```python
from build123d import *

# Parameters (mm, degrees)
F0_W     = 10
F0_H     = 13
F1_DEPTH = 32
F2_R     = 5.5
F3_DEPTH = 25
F4_R     = 6.5
F5_DEPTH = 25
F7_DEPTH = 19


with BuildPart() as f1:
    # F0 (on Front) → F1 (new body)
    with BuildSketch(Plane.XZ):
        with Locations((-52.5, -6.5)):
            Rectangle(F0_W, F0_H)
        Polygon((-47.5, 0), (-47.5, -13), (-18.5, -13), (-18.5, 0), (0, 0), (0, 13), (-13.5, 13), (-13.5, 51), (-32.5, 51), (-32.5, 0), align=None)
    extrude(amount=-F1_DEPTH)

    # F2 (on face) → F3 (cut)
    with BuildSketch(Plane.XY):
        with Locations((-45, 19)):
            Circle(F2_R)
        Polygon((-57.5, 0), (-47.5, 0), (-57.5, 10), align=None)
    extrude(amount=-F3_DEPTH, mode=Mode.SUBTRACT)

    # F4 (on face) → F5 (cut)
    with BuildSketch(Plane.YZ.offset(-13.5)):
        with Locations((16, 33)):
            Circle(F4_R)
    extrude(amount=-F5_DEPTH, mode=Mode.SUBTRACT)

    # F6 (on face) → F7 (join)
    with BuildSketch(Plane.YZ.offset(-13.5)):
        with BuildLine():
            Line((0, 51), (32, 51))
            ThreePointArc((32, 51), (16, 54.871235), (0, 51))
        make_face()
    extrude(amount=-F7_DEPTH)

    # F8: F1 across plane


with BuildPart() as f1_1:
    add(f1.part)
    add(f1.part.mirror(Plane.YZ))


solid = f1_1.part
```
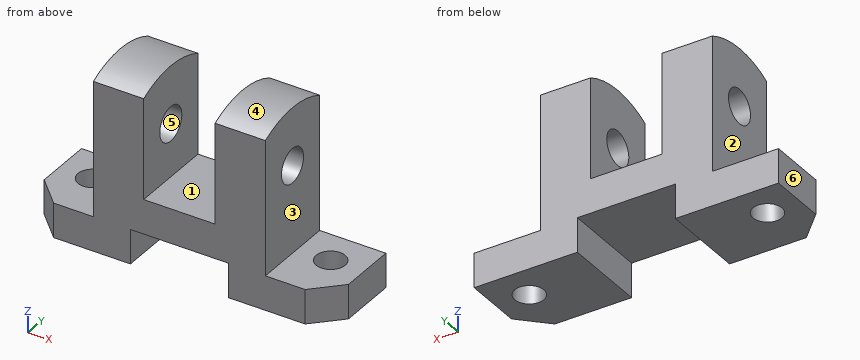
Could you check a few things on this model? Use its own coordinates, in mm. Face numbers are marked on the shaded views. A direction names the side the tool comes from. Coordinates: 2 decimals unless noted, no trailing zeros. Write each loop counter-clockwise with the first axis right and the second up, starting at its lowest first coordinate (ties: lowest second). Pieces come first, ordered by that corner, then holes. Notation, with made-up numbers: (35, -8) - (91, -8) arc R13 ccw to (91, 7) - close; hole circle Ø9 at (-34, 58). An arc over 180 degrees is marked (long way). Use a Markdown table: item, result.
Q1. Imagine slicing it at A-A (z = 33). List the corners of the cut face in (x, y) for me, and give its area (3 significant figures).
Geometry check:
| item | result |
|---|---|
| outline | (-32.5, 0) - (-13.5, 0) - (-13.5, 9.5) - (-32.5, 9.5) - close; (-32.5, 22.5) - (-13.5, 22.5) - (-13.5, 32) - (-32.5, 32) - close; (13.5, 0) - (32.5, 0) - (32.5, 9.5) - (13.5, 9.5) - close; (13.5, 22.5) - (32.5, 22.5) - (32.5, 32) - (13.5, 32) - close |
| area | 722 mm2 |
Q2. I'm going to push flat-ended pins straight in: pin 1 Ø17.5 at (x, y) = (45, 19) entering from +Z; pin 2 Ø13.5 at (x, y) = (6, 15) entering from +Z; pin 3 Ø16 at (y, z) = (19, 35) entering from +X. Where does each tip first touch, or does it pass through?
Geometry check:
| item | result |
|---|---|
| pin 1 | stops at z = 0 |
| pin 2 | stops at z = 13 |
| pin 3 | stops at x = 32.5 |
Q3. Imagine slicing it at D-D (x = 20.5). List the corners of the cut face in (y, z) for me, and give its area (3 significant figures).
Geometry check:
| item | result |
|---|---|
| outline | (0, -13) - (32, -13) - (32, 51) arc R35 ccw to (0, 51) - close; hole circle Ø13 at (16, 33) |
| area | 2,000 mm2 |
Q4. Imagine slicing it at B-B (x = -45). List the corners of the cut face in (y, z) for me, and give its area (3 significant figures).
Geometry check:
| item | result |
|---|---|
| outline | (0, -13) - (13.5, -13) - (13.5, 0) - (0, 0) - close; (24.5, -13) - (32, -13) - (32, 0) - (24.5, 0) - close |
| area | 273 mm2 |
Q5. Which directions (+Z, -Z, +X, -X, +Y, -Y) give clear straight access to the entire face, cutting with the end or side of a thin tool? Please do the marked faces 1, 2 and 3.
Geometry check:
| item | result |
|---|---|
| face 1 | +Z, +Y, -Y |
| face 2 | +Z, -X, +Y, -Y |
| face 3 | +Z, +X, +Y, -Y |
Q6. Imagine slicing it at C-C (y = 15). Count the separate pieces of the cut face and the enclosed holes in it, and give its area (3 significant figures).
Geometry check:
| item | result |
|---|---|
| separate pieces | 5 |
| enclosed holes | 0 |
| area | 2,770 mm2 |
Q7. Please list where these lines run through material, in increasing order: L1, parallel to Y at x = -45, z = -5; L2, parallel to X at y = 20, z = 14; L3, parallel to Z at x = 42, y = 26.5.
Geometry check:
| item | result |
|---|---|
| L1 | y = 0 to 13.5, 24.5 to 32 |
| L2 | x = -32.5 to -13.5, 13.5 to 32.5 |
| L3 | z = -13 to 0 |
Q8. Thinking about a two-plate mould opening in Z: for the marked faces 4, 5 and 6, which applies, +Z half, -Z half, draft (parallel to the pull), parting line (faces both ways), or undercut?
Geometry check:
| item | result |
|---|---|
| face 4 | +Z half |
| face 5 | undercut |
| face 6 | draft |
